Part model, mm, in its own coordinate system. Round coordinates to 2 decimals unless told otherwise and drop trailing zeros. Loops run counter-clockwise (first coordinate to the right, second up) from the corner with the lowest first, then second, coordinate; pieces in that order, holes last. Notation, with made-up numbers: (-16, 32) - (33, 32) arc R8 cw to (33, 37) - close; hole circle Ø8 at (70, -9). An arc over 180 degrees is marked (long way). Put each result on its own line as item: value.
from build123d import *

# Parameters (mm, degrees)
SKETCH1_W                    = 287
SKETCH1_H                    = 175
BASE_FLANGE1_DEPTH           = 1
EDGE_FLANGE1_STRIP_W         = 5.4732
EDGE_FLANGE1_STRIP_H         = 1
EDGE_FLANGE1_STRIP_CUT_DEPTH = 175
EDGE_FLANGE1_DEPTH           = 175
EDGE_FLANGE2_STRIP_W         = 5.4732
EDGE_FLANGE2_STRIP_H         = 1
EDGE_FLANGE2_STRIP_CUT_DEPTH = 463.2634
EDGE_FLANGE2_DEPTH           = 463.2634
SKETCH17_R                   = 4.794
SKETCH17_R_2                 = 2.794
BOSS_EXTRUDE1_DEPTH          = 18
SKETCH21_R                   = 5
SKETCH21_R_2                 = 3
BOSS_EXTRUDE2_DEPTH          = 5


# Sheet-metal steps are written as plain solids
with BuildPart() as part:
    # Sketch1 → Base-Flange1 (new body)
    with BuildSketch(Plane.XY):
        Rectangle(SKETCH1_W, SKETCH1_H)
    extrude(amount=-BASE_FLANGE1_DEPTH)

    # Edge-Flange1 strip (across the edge) → Edge-Flange1 strip cut (cut)
    with BuildSketch(Plane(origin=(-143.5, -87.5, -1), x_dir=(1, 0, 0), z_dir=(0, 1, 0))):
        with Locations((-1, -0.5)):
            Rectangle(EDGE_FLANGE1_STRIP_W, EDGE_FLANGE1_STRIP_H)
    extrude(amount=EDGE_FLANGE1_STRIP_CUT_DEPTH, mode=Mode.SUBTRACT)

    # Edge-Flange1 section (across the edge) → Edge-Flange1 (add)
    with BuildSketch(Plane(origin=(-143.5, -87.5, -1), x_dir=(1, 0, 0), z_dir=(0, 1, 0))):
        with BuildLine():
            Line((0, 0.7366), (0, 464))
            Line((0, 464), (1, 464))
            Line((1, 464), (1, 0.7366))
            ThreePointArc((1, 0.7366), (1.215745145, 0.215745145), (1.7366, 0))
            Line((1.7366, 0), (1.7366, -1))
            ThreePointArc((1.7366, -1), (0.508638364, -0.491361636), (0, 0.7366))
        make_face()
    extrude(amount=EDGE_FLANGE1_DEPTH)

    # Edge-Flange2 strip (across the edge) → Edge-Flange2 strip cut (cut)
    with BuildSketch(Plane(origin=(-143.5, 87.5, -1.7366), x_dir=(0, -1, 0), z_dir=(0, 0, -1))):
        with Locations((-1, -0.5)):
            Rectangle(EDGE_FLANGE2_STRIP_W, EDGE_FLANGE2_STRIP_H)
    extrude(amount=EDGE_FLANGE2_STRIP_CUT_DEPTH, mode=Mode.SUBTRACT)

    # Edge-Flange2 section (across the edge) → Edge-Flange2 (add)
    with BuildSketch(Plane(origin=(-143.5, 87.5, -1.7366), x_dir=(0, -1, 0), z_dir=(0, 0, -1))):
        with BuildLine():
            Line((0, 0.7366), (0, 17))
            Line((0, 17), (1, 17))
            Line((1, 17), (1, 0.7366))
            ThreePointArc((1, 0.7366), (1.215745145, 0.215745145), (1.7366, 0))
            Line((1.7366, 0), (1.7366, -1))
            ThreePointArc((1.7366, -1), (0.508638364, -0.491361636), (0, 0.7366))
        make_face()
    extrude(amount=EDGE_FLANGE2_DEPTH)

    # Sketch17 → Boss-Extrude1 (add)
    # profile 1 of 4: a face of its own
    with BuildSketch(Plane.ZY.offset(143.5)):
        with Locations((-72.584668807, 78.453866984)):
            Circle(SKETCH17_R)
        with Locations((-72.584668807, 78.453866984)):
            Circle(SKETCH17_R_2, mode=Mode.SUBTRACT)
    # profile 2 of 4: a face of its own
    with BuildSketch(Plane.ZY.offset(143.5)):
        with Locations((-182.592068807, 78.453866984)):
            Circle(SKETCH17_R)
        with Locations((-182.592068807, 78.453866984)):
            Circle(SKETCH17_R_2, mode=Mode.SUBTRACT)
    # profile 3 of 4: a face of its own
    with BuildSketch(Plane.ZY.offset(143.5)):
        with Locations((-292.599468807, 78.453866984)):
            Circle(SKETCH17_R)
        with Locations((-292.599468807, 78.453866984)):
            Circle(SKETCH17_R_2, mode=Mode.SUBTRACT)
    # profile 4 of 4: a face of its own
    with BuildSketch(Plane.ZY.offset(143.5)):
        with Locations((-402.606868807, 78.453866984)):
            Circle(SKETCH17_R)
        with Locations((-402.606868807, 78.453866984)):
            Circle(SKETCH17_R_2, mode=Mode.SUBTRACT)
    extrude(amount=BOSS_EXTRUDE1_DEPTH)

    # Sketch21 → Boss-Extrude2 (add)
    # profile 1 of 2: a face of its own
    with BuildSketch(Plane.XY):
        with Locations(Location((81.5, 52.5, 0), (0, 0, 180))):
            Circle(SKETCH21_R)
        with Locations((81.5, 52.5)):
            Circle(SKETCH21_R_2, mode=Mode.SUBTRACT)
    # profile 2 of 2: a face of its own
    with BuildSketch(Plane.XY):
        with Locations(Location((81.5, -7.5, 0), (0, 0, 180))):
            Circle(SKETCH21_R)
        with Locations((81.5, -7.5)):
            Circle(SKETCH21_R_2, mode=Mode.SUBTRACT)
    extrude(amount=BOSS_EXTRUDE2_DEPTH)


solid = part.part
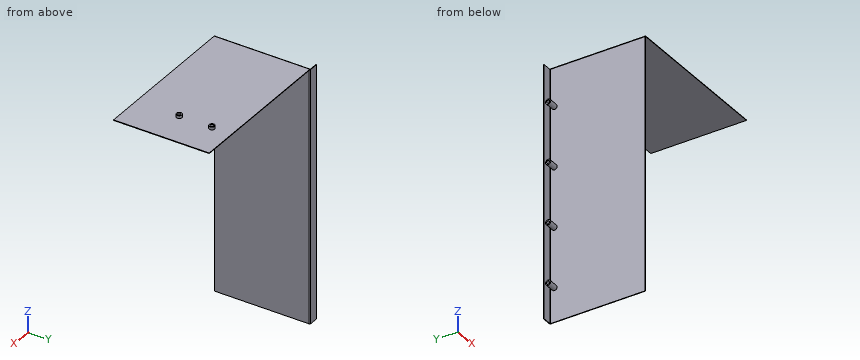
1. Pin check, flat tips, straight feed: P1, Ø1.1, axis at y = 87, z = -125.5, coming from the -X side; P2, Ø6, axis at y = 63, z = -196, coming from the +X side; P3, Ø1.9, axis at x = -156, y = 86.5, coming from the +Z side. Stop position of each tip, or through.
A:
P1: stops at x = -160.5
P2: stops at x = -142.5
P3: stops at z = -1.74
2. Probe line 1 along X through (y, z) = (-7, 1); line 2 along Y through (x, z) = (81.5, 3.4); line 3 along Z through (x, y) = (16, -24). List the from-to ranges inside material, lowest first. Write a range as [from, to].
A:
line 1: x = [76.53, 78.54], [84.46, 86.47]
line 2: y = [-12.5, -10.5], [-4.5, -2.5], [47.5, 49.5], [55.5, 57.5]
line 3: z = [-1, 0]
3. Band-saw the part on C-C (x = -90). List the corners of the cut face in (y, z).
A:
outline: (-87.5, -1) - (87.5, -1) - (87.5, 0) - (-87.5, 0) - close
4. Band-saw the part on A-A (z = -355.5). List the corners of the cut face in (x, y), plus the area to 3 significant figures.
A:
outline: (-160.5, 86.5) - (-144.24, 86.5) arc R0.74 cw to (-143.5, 85.76) - (-143.5, -87.5) - (-142.5, -87.5) - (-142.5, 85.76) arc R1.74 ccw to (-144.24, 87.5) - (-160.5, 87.5) - close
area: 191 mm²
5. Band-saw the part on B-B (y = -54.5). List the corners of the cut face in (x, z).
A:
outline: (-143.5, -465) - (-142.5, -465) - (-142.5, -1.74) arc R0.74 cw to (-141.76, -1) - (143.5, -1) - (143.5, 0) - (-141.76, 0) arc R1.74 ccw to (-143.5, -1.74) - close
